For this review, use the dimensioned drawing (mm, ordinates from the lowest corner) and the shaded views. Coordinates: 2 decimals unless noted, no trailing zeros. Write each loop counter-clockwise with the first axis right and the second up, starting at its lowest first coordinate (ties: lowest second). Pieces come first, ordered by that corner, then holes. Notation, with made-up numbers: (1, 51.5) - (15, 51.5) arc R14 cw to (15, 78.5) - close; hole circle Ø3 at (56, 17). An arc over 180 degrees is marked (long way). One line per item, written item: value.
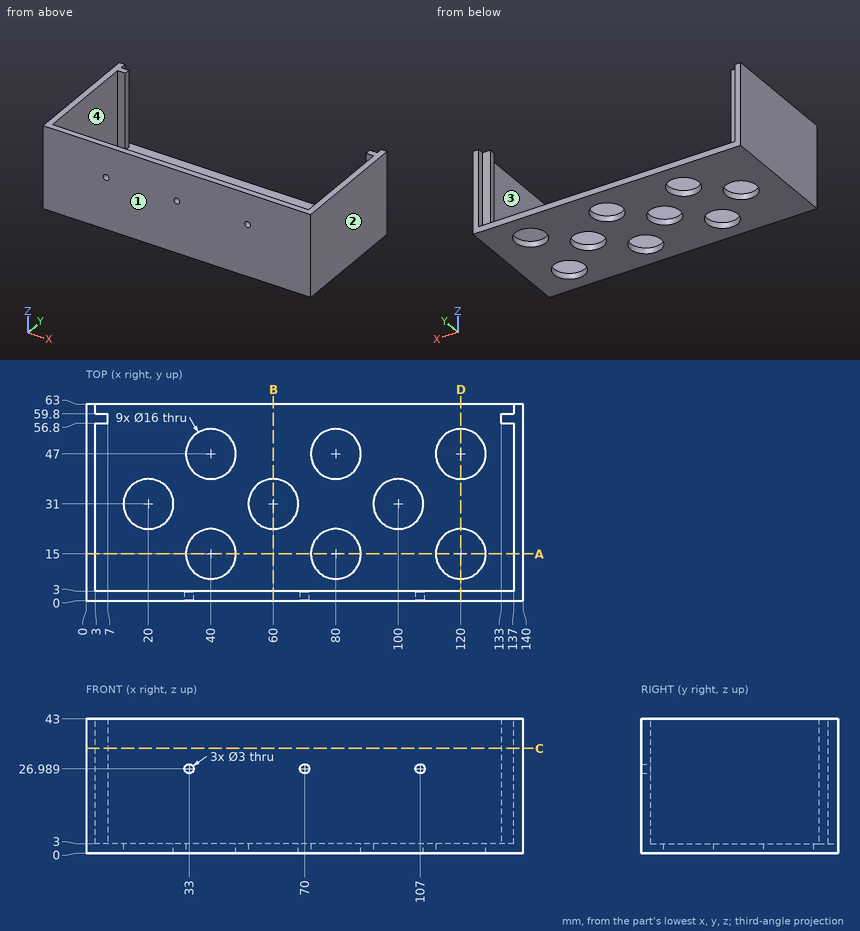
1. Consider section D-D, the plane x = 120. Write out the cut boundary in (y, z), then the cut area to 3 significant figures.
Answer block:
outline: (0, 0) - (7, 0) - (7, 3) - (3, 3) - (3, 43) - (0, 43) - close; (23, 0) - (39, 0) - (39, 3) - (23, 3) - close; (55, 0) - (63, 0) - (63, 3) - (55, 3) - close
area: 213 mm^2
2. Mouldability with a two-part tool opening along Y and no side actions: class the marked faces 1, 2, 3 and 4 as released by +Y, released by -Y, zero draft, split by the parting line, or undercut.
Answer block:
face 1: released by -Y
face 2: zero draft
face 3: undercut
face 4: undercut
3. Consider section C-C, the plane z = 33.5. Write out the cut boundary in (x, y), then the cut area to 3 significant figures.
Answer block:
outline: (0, 0) - (140, 0) - (140, 63) - (137, 63) - (137, 59.8) - (133, 59.8) - (133, 56.8) - (137, 56.8) - (137, 3) - (3, 3) - (3, 56.8) - (7, 56.8) - (7, 59.8) - (3, 59.8) - (3, 63) - (0, 63) - close
area: 804 mm^2
4. Wall thickness on line 1 along X through (y, z) = (32.5, 33); line 2 along Y through (x, z) = (40, 0.75); line 3 along Z through (x, y) = (33, 1.8): over which ranges is each line inside the solid? List them lowest first.
Answer block:
line 1: x = 0 to 3, 137 to 140
line 2: y = 0 to 7, 23 to 39, 55 to 63
line 3: z = 0 to 25.49, 28.49 to 43
5. Insertion check: pin 1 Ø18.5 at (x, y) = (40, 15) entering from +Z; pin 2 Ø10 at (x, z) = (117.5, 9.5) entering from +Y; pin 3 Ø1.2 at (x, z) = (135, 22.5) entering from +Y. Each pin has a flat end and moves straight along its axis. Give the tip position at first contact, or say it passes through.
Answer block:
pin 1: stops at z = 3
pin 2: stops at y = 3
pin 3: stops at y = 59.8
6. Consider section A-A, the plane y = 15. Write out the cut boundary in (x, z).
Answer block:
outline: (0, 0) - (32, 0) - (32, 3) - (3, 3) - (3, 43) - (0, 43) - close; (48, 0) - (72, 0) - (72, 3) - (48, 3) - close; (88, 0) - (112, 0) - (112, 3) - (88, 3) - close; (128, 0) - (140, 0) - (140, 43) - (137, 43) - (137, 3) - (128, 3) - close
7. Consider section B-B, the plane x = 60. Write out the cut boundary in (y, z), then the cut area to 3 significant figures.
Answer block:
outline: (0, 0) - (23, 0) - (23, 3) - (3, 3) - (3, 43) - (0, 43) - close; (39, 0) - (63, 0) - (63, 3) - (39, 3) - close
area: 261 mm^2
